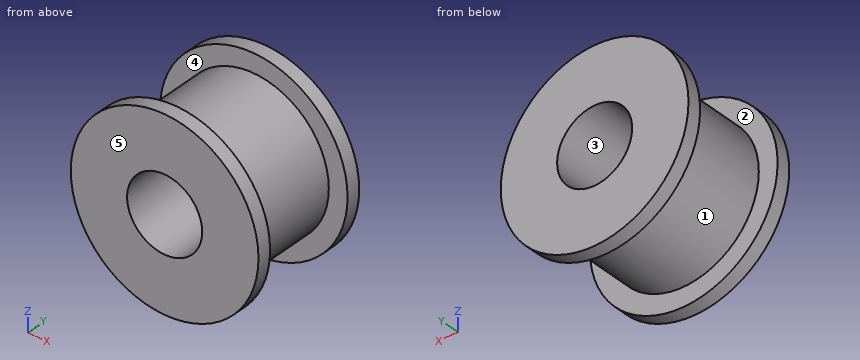
from build123d import *

# Parameters (mm, degrees)
F0_R     = 10
F1_DEPTH = 1.5
F2_R     = 8
F3_DEPTH = 10
F4_R     = 10
F5_DEPTH = 1.5
F6_R     = 4
F7_DEPTH = 25


with BuildPart() as f1:
    # F0 (on Front) → F1 (new body)
    with BuildSketch(Plane.XZ):
        Circle(F0_R)
    extrude(amount=F1_DEPTH)

    # F2 (on face) → F3 (join)
    with BuildSketch(Plane.XZ.offset(1.5)):
        Circle(F2_R)
    extrude(amount=F3_DEPTH)

    # F4 (on face) → F5 (join)
    with BuildSketch(Plane.XZ.offset(11.5)):
        Circle(F4_R)
    extrude(amount=F5_DEPTH)

    # F6 (on face) → F7 (cut)
    with BuildSketch(Plane.XZ.offset(13)):
        Circle(F6_R)
    extrude(amount=-F7_DEPTH, mode=Mode.SUBTRACT)


solid = f1.part
Source: CAD feature listing. Evaluate the final solid. Frame: model axes, mm. Face numbers are marked on the shaded views. A direction names the side the tool comes from. Round coordinates to 2 decimals unless told otherwise and drop trailing zeros. Loops run counter-clockwise (first coordinate to the right, second up) from the corner with the lowest first, then second, coordinate; pieces in that order, holes last. Notation, with made-up numbers: M 17,67 L 50,67 A22 cw 50,94 Z; hole C -11,-25 d2. An arc over 180 degrees is marked long. Return JSON: item names as keys, results as strings. Group by question number.
1. Section query C-C on y = -2.25. Output: boundary loops of the cut face in (x, z).
2. Section query B-B on z = 0. Output: boundary loops of the cut face in (x, y), and give its area (3 significant figures).
3. Pin query (flat end, axial travel): pin 1 (2 mm diameter, centred on y = -11, z = -3.5, fed in from +X); pin 2 (5 mm diameter, centred on x = 4, y = -2.5, fed in from +Z). Return the tip coordinate at first contact, or that it passes through.
4. Mould query, pull axis X, two halves, no side actions, for the marked faces 1, 2 and 3. Classes: released by +X, released by -X, zero draft, split by the parting line, or undercut.
5. Section query D-D on z = -7.25. Output: boundary loops of the cut face in (x, y).
6. Reachability of the marked faces 4 and 5 from +Z, -Z, +X, -X, +Y, -Y: full face, straight path, thin tool, end or side. Return the list, or none.
7. Material intervals for line 1 along Y through (x, z) = (-4, -7); line 2 along Z through (x, y) = (0, -5.25); line 3 along Z through (x, y) = (-2.75, -5.5), sorted ascending. Write a range as from..to.
8. Section query A-A on x = 0. Output: boundary loops of the cut face in (y, z).
Checks:
{
 "1": {"outline": "C 0,0 d16; hole C 0,0 d8"},
 "2": {"outline": "M -10,-13 L -4,-13 L -4,0 L -10,0 L -10,-1.5 L -8,-1.5 L -8,-11.5 L -10,-11.5 Z; M 4,-13 L 10,-13 L 10,-11.5 L 8,-11.5 L 8,-1.5 L 10,-1.5 L 10,0 L 4,0 Z", "area": "116 mm²"},
 "3": {"pin 1": "stops at x = 9.65", "pin 2": "stops at z = 9.85"},
 "4": {"face 1": "split by the parting line", "face 2": "zero draft", "face 3": "undercut"},
 "5": {"outline": "M -6.89,-13 L 6.89,-13 L 6.89,-11.5 L 3.38,-11.5 L 3.38,-1.5 L 6.89,-1.5 L 6.89,0 L -6.89,0 L -6.89,-1.5 L -3.38,-1.5 L -3.38,-11.5 L -6.89,-11.5 Z"},
 "6": {"face 4": "none", "face 5": "+Z, -Z, +X, -X, -Y"},
 "7": {"line 1": "y = -13..-11.5, -1.5..0", "line 2": "z = -8..-4, 4..8", "line 3": "z = -7.51..-2.9, 2.9..7.51"},
 "8": {"outline": "M -13,-10 L -11.5,-10 L -11.5,-8 L -1.5,-8 L -1.5,-10 L 0,-10 L 0,-4 L -13,-4 Z; M -13,4 L 0,4 L 0,10 L -1.5,10 L -1.5,8 L -11.5,8 L -11.5,10 L -13,10 Z"}
}
